Geometry check sheet. Reference: the model listing, model coordinates, mm. Face numbers are marked on the shaded views. A direction names the side the tool comes from. Coordinates: 2 decimals unless noted, no trailing zeros. Write each loop counter-clockwise with the first axis right and the second up, starting at its lowest first coordinate (ties: lowest second). Pieces come first, ordered by that corner, then holes. Notation, with made-up numbers: (8.5, 76) -> (45.5, 76) arc R31 ccw to (45.5, 103) -> close; hole circle Ø11 at (-22, 35.5). An arc over 180 degrees is marked (long way). Put each result on its own line as item: value. Start each with the question number.
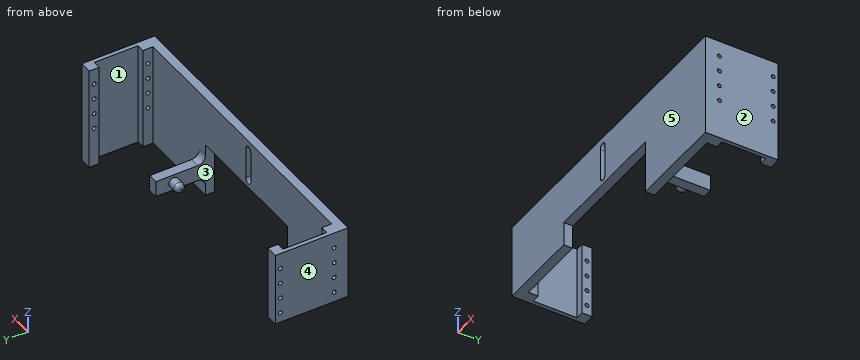
Autodesk Fusion 360 part; units mm, degrees
sketch "Sketch1" plane through (0, 0, 0) normal (0, 0, 1) x (1, 0, 0)
  line L0 (0, 0) -> (144.5, 0)
  line L1 (0, 0) -> (0, 5)
  line L2 (144.5, 0) -> (144.5, 5)
  line L3 (0, 5) -> (-4, 5)
  line L4 (144.5, 5) -> (148.5, 5)
  line L5 (-4, 5) -> (-4, 27)
  line L6 (-4, 27) -> (0, 27)
  line L7 (0, 27) -> (0, 32)
  line L8 (148.5, 5) -> (148.5, 27)
  line L9 (148.5, 27) -> (144.5, 27)
  line L10 (144.5, 27) -> (144.5, 32)
  line L11 (0, 32) -> (-6, 32)
  line L12 (-6, 32) -> (-6, -3)
  line L13 (-6, -3) -> (150.5, -3)
  line L14 (150.5, -3) -> (150.5, 32)
  line L15 (150.5, 32) -> (144.5, 32)
  dimension "d2" = 5
  dimension "d3" = 5
  dimension "d4" = 4
  dimension "d5" = 4
  dimension "d6" = 22
  dimension "d7" = 22
  dimension "d8" = 5
  dimension "d10" = 6
  dimension "d11" = 35
  dimension "d12" = 156.5
  dimension "d13" = 35
  dimension "d83" = 2
  dimension "d84" = 2
  dimension "d85" = 6
  dimension "d86" = 6
  dimension "d87" = 6
extrude "Extrude1" add sketch "Sketch1" along normal blind 37
sketch "Sketch2" plane through (-6, 0, 0) normal (-1, 0, 0) x (0, -1, 0)
  line L0 (-32, 0) -> (3, 0)
  line L1 (3, 0) -> (3, 37)
  line L2 (3, 37) -> (-32, 37)
  line L3 (-32, 37) -> (-32, 0)
  line L4 (-27, 37) -> (-32, 37)
  circle A0 centre (-29.5, 5) radius 1
  circle A1 centre (-29.5, 13) radius 1
  circle A2 centre (-29.5, 21) radius 1
  circle A3 centre (-29.5, 29) radius 1
  circle A4 centre (-2.5, 29) radius 1
  circle A5 centre (-2.5, 21) radius 1
  circle A6 centre (-2.5, 13) radius 1
  circle A7 centre (-2.5, 5) radius 1
  dimension "d18" = 2
  dimension "d19" = 2
  dimension "d21" = 2
  dimension "d22" = 8
  dimension "d24" = 8
  dimension "d25" = 2
  dimension "d26" = 8
hole "Hole2" at (-6, 2.5, 29) at (-6, 2.5, 21) at (-6, 2.5, 13) at (-6, 2.5, 5) direction (1, 0, 0) diameter 2 depth 80 tip angle 118
hole "Hole3" at (-6, 29.5, 29) direction (1, 0, 0) diameter 2 depth 280 tip angle 118
hole "Hole4" at (-6, 29.5, 21) at (-6, 29.5, 13) at (-6, 29.5, 5) at (-6, 2.5, 29) at (-6, 2.5, 21) at (-6, 2.5, 13) at (-6, 2.5, 5) direction (1, 0, 0) diameter 2 depth 245 tip angle 118
sketch "Sketch3" plane through (0, -3, 0) normal (0, -1, 0) x (1, 0, 0)
  line L0 (-6, 0) -> (150.5, 0)
  line L1 (150.5, 0) -> (150.5, 37)
  line L2 (150.5, 37) -> (-6, 37)
  line L3 (-6, 37) -> (-6, 0)
  line L4 (36, 0) -> (36, 12)
  line L5 (36, 12) -> (102, 12)
  line L6 (102, 12) -> (102, 0)
  line L7 (36, 0) -> (102, 0)
  line L8 (-6, 0) -> (-6, 37)
  dimension "d45" = 12
  dimension "d79" = 12
  dimension "d81" = 42
  dimension "d82" = 66
extrude "Extrude2" cut sketch "Sketch3" against normal blind 9 contours L0 L4 L5 L6 L7
sketch "Sketch4" plane through (150.5, 0, 0) normal (1, 0, 0) x (0, 1, 0)
  line L0 (-3, 0) -> (32, 0)
  line L1 (32, 0) -> (32, 37)
  line L2 (32, 37) -> (-3, 37)
  line L3 (-3, 37) -> (-3, 0)
  circle A0 centre (14.5, 44) radius 2.1
  line L4 (14.5, 49.1) -> (10, 49.1)
  line L5 (10, 49.1) -> (10, 37)
  line L6 (19, 49.1) -> (19, 37)
  line L7 (19, 37) -> (14.5, 37)
  line L8 (19, 49.1) -> (14.5, 49.1)
  circle A1 centre (2.5, 13) radius 1
  circle A2 centre (2.5, 29) radius 1
  circle A3 centre (29.5, 13) radius 1
  circle A4 centre (29.5, 21) radius 1
  circle A5 centre (29.5, 5) radius 1
  circle A6 centre (2.5, 21) radius 1
  circle A7 centre (2.5, 5) radius 1
  circle A8 centre (29.5, 29) radius 1
  dimension "d46" = 17.5
  dimension "d47" = 7
  dimension "d48" = 4.2
sketch "Sketch5" plane through (150.5, 0, 0) normal (1, 0, 0) x (0, 1, 0)
  line L0 (32, 37) -> (-3, 37)
  line L1 (-3, 37) -> (-3, 0)
  line L2 (-3, 0) -> (32, 0)
  line L3 (32, 0) -> (32, 37)
  line L4 (6.9, 0) -> (6.9, 10)
  line L5 (22.1, 0) -> (22.1, 37)
  line L6 (22.1, 0) -> (24.1, 0)
  line L7 (24.1, 0) -> (24.1, 37)
  line L8 (6.9, 0) -> (4.9, 0)
  line L9 (4.9, 0) -> (4.927, 10.0053)
  line L10 (6.9, 0) -> (6.9, 10)
  line L11 (6.9, 10) -> (4.9, 10.0054)
  circle A0 centre (2.5, 13) radius 1
  circle A1 centre (2.5, 29) radius 1
  circle A2 centre (29.5, 13) radius 1
  circle A3 centre (29.5, 21) radius 1
  circle A4 centre (29.5, 5) radius 1
  circle A5 centre (2.5, 21) radius 1
  circle A6 centre (2.5, 5) radius 1
  circle A7 centre (29.5, 29) radius 1
  point P0 (5, 37)
  point P1 (5, 37)
  dimension "d54" = 9.9
  dimension "d55" = 9.9
  dimension "d56" = 2
  dimension "d57" = 2
  dimension "d60" = 10
  dimension "d61" = 2
ref_plane "WorkPlane1" through (102.5, 14.5, 18.5) normal (1, 0, 0) x (0, 1, 0)
sketch "Sketch7" plane through (0, -3, 0) normal (0, -1, 0) x (1, 0, 0)
  line L0 (36, 0) -> (36, 12)
  line L1 (36, 12) -> (102, 12)
  line L2 (102, 12) -> (102, 0)
  line L3 (102, 0) -> (150.5, 0)
  line L4 (150.5, 0) -> (150.5, 37)
  line L5 (150.5, 37) -> (-6, 37)
  line L6 (-6, 37) -> (-6, 0)
  line L7 (-6, 0) -> (36, 0)
  line L8 (65.5, 32) -> (65.5, 16)
  line L9 (69.5, 32) -> (69.5, 16)
  arc A0 (69.5, 32) -> (65.5, 32) centre (67.5, 32) ccw
  arc A1 (65.5, 16) -> (69.5, 16) centre (67.5, 16) ccw
  dimension "d71" = 4
  dimension "d74" = 4
  dimension "d76" = 2
  dimension "d88" = 71.5
  dimension "d89" = 4
extrude "Extrude7" cut sketch "Sketch7" against normal blind 13 contours L8 L9 A0 A1
extrude "Extrude8" add 1 faces at (134.3333, -3, 16.3333) along direction (0, -1, 0) blind 1.5
extrude "Extrude9" add 1 faces at (132.3333, -3, 0) along direction (0, 0, -1) blind 15
sketch "Sketch8" plane through (0, 0, 0) normal (0, 1, 0) x (-1, 0, 0)
  line L0 (-65.5, 32) -> (-65.5, 16)
  arc A0 (-69.5, 16) -> (-65.5, 16) centre (-67.5, 16) ccw
  line L1 (-69.5, 16) -> (-69.5, 32)
  arc A1 (-65.5, 32) -> (-69.5, 32) centre (-67.5, 32) ccw
  line L2 (-36, 12) -> (-36, 0)
  line L3 (-36, 0) -> (0, 0)
  line L4 (0, 0) -> (0, 37)
  line L5 (0, 37) -> (-144.5, 37)
  line L6 (-144.5, 37) -> (-144.5, -15)
  line L7 (-144.5, -15) -> (-102, -15)
  line L8 (-102, -15) -> (-102, 12)
  line L9 (-102, 12) -> (-36, 12)
  line L10 (-102, 2.5) -> (-107, 2.5)
  line L11 (-102, -5.5) -> (-107, -5.5)
  line L12 (-107, -5.5) -> (-107, 2.5)
  line L13 (-102, 2.5) -> (-102, -5.5)
  dimension "d97" = 5
  dimension "d100" = 8
  dimension "d101" = 8
  dimension "d102" = 9.5
extrude "Extrude10" add sketch "Sketch8" along normal blind 25 contours L8 L10 L11 L12 L13
sketch "Sketch10" plane through (102, 0, 0) normal (-1, 0, 0) x (0, -1, 0)
  line L0 (0, -5.5) -> (0, -15)
  line L1 (0, -15) -> (4.5, -15)
  line L2 (4.5, -15) -> (4.5, 12)
  line L3 (4.5, 12) -> (0, 12)
  line L4 (0, 12) -> (0, 2.5)
  line L5 (0, 2.5) -> (-25, 2.5)
  line L6 (-25, 2.5) -> (-25, -5.5)
  line L7 (-25, -5.5) -> (0, -5.5)
  circle A0 centre (-16, -1.5) radius 2.5
  dimension "d107" = 5
  dimension "d108" = 9
extrude "Extrude12" add sketch "Sketch10" along normal blind 6 contours A0
fillet "Fillet4" radius 2 1 edges at (96, 18.3308, -2.404)
fillet "Fillet5" radius 4 2 edges at (104.5, 0, -5.5) (104.5, 0, 2.5)
equation "d11 = 32.00 mm + 3 mm"
equation "d12 = 96 mm + 10.5 mm + 50 mm"
equation "d46 = ( 35 / 2 ) * 1 mm"
equation "d64 = ( -96 / 2 ) * 1 mm"
equation "d88 = 46.50 mm + 25 mm"
Item 1: Section check C-C, the plane x = 21.5. Enter the section's corners in (y, z).
Item 2: Section check A-A, the plane z = 26. Enter the section's corners in (x, y), and give its area (3 significant figures).
Item 3: Section check B-B, the plane x = 135. Enter the section's corners in (y, z), and give its area (3 significant figures).
Item 4: Access from +Z, -Z, +X, -X, +Y, -Y to the whole of each face (thin tool, end or side, straight path). Record for the marked faces 1 and 2.
Item 5: Mould release check, pull along X, two halves, no side actions. Record for the marked faces 3, 4 and 5: released by +X, released by -X, zero draft, split by the parting line, or undercut.
Item 6: Go/stop test with flat-tipped pins: P1, Ø1.8, axis at y = 29.5, z = 5, coming from the +X side; P2, Ø2.5, axis at y = 29.5, z = 13, coming from the -X side; P3, Ø12, axis at x = 119.5, z = 31, coming from the +Y side; P4, Ø4, axis at x = 53.5, y = 0.5, coming from the -Z side. Record where each tip stops, or that it passes through.
Item 7: Scan lines: line 1 along Z through (x, y) = (-1.9, 29.5); line 2 along Z through (x, y) = (146.15, 2.5); line 3 along Y through (x, z) = (146, 13). Record each from-to range of solid material in increasing order. Write a range as [from, to].
From the geometry:
1. outline: (-4.5, 0) -> (0, 0) -> (0, 37) -> (-4.5, 37) -> close
2. outline: (-6, -4.5) -> (65.5, -4.5) -> (65.5, 0) -> (0, 0) -> (0, 5) -> (-4, 5) -> (-4, 27) -> (0, 27) -> (0, 32) -> (-6, 32) -> close; (69.5, -4.5) -> (150.5, -4.5) -> (150.5, 32) -> (144.5, 32) -> (144.5, 27) -> (148.5, 27) -> (148.5, 5) -> (144.5, 5) -> (144.5, 0) -> (69.5, 0) -> close
2. area: 894 mm²
3. outline: (-4.5, -15) -> (0, -15) -> (0, 37) -> (-4.5, 37) -> close
3. area: 234 mm²
4. face 1: +Z, -Z
4. face 2: +Z, -Z, +X, +Y, -Y
5. face 3: undercut
5. face 4: released by -X
5. face 5: zero draft
6. P1: through
6. P2: x = -6
6. P3: y = 0
6. P4: z = 12
7. line 1: [0, 4], [6, 12], [14, 20], [22, 28], [30, 37]
7. line 2: [-15, 4], [6, 12], [14, 20], [22, 28], [30, 37]
7. line 3: [-4.5, 1.5], [3.5, 5], [27, 28.5], [30.5, 32]
